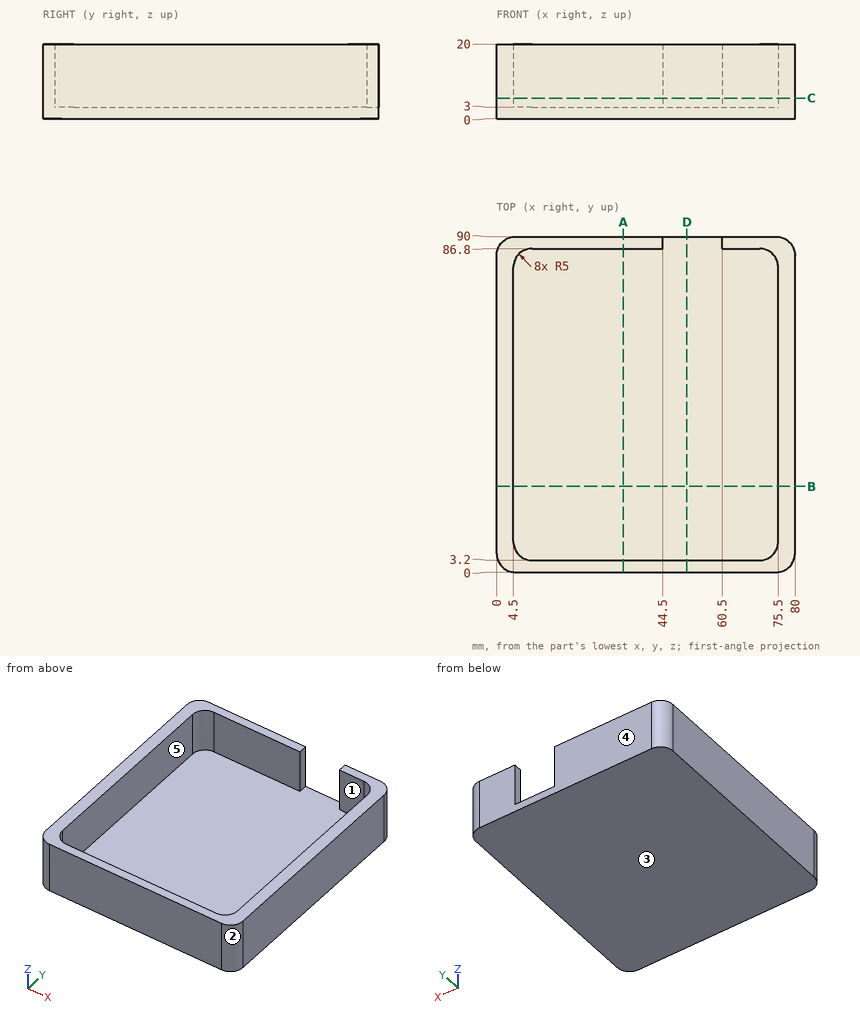
Source: three-view drawing plus pictorial views. Frame: mm from the lowest corner of the part. A direction names the side the tool comes from. Coordinates: 2 decimals unless noted, no trailing zeros. Loops run counter-clockwise (first coordinate to the right, second up) from the corner with the lowest first, then second, coordinate; pieces in that order, holes last. Notation, with made-up numbers: (59, 34) - (64, 34) arc R25 cw to (64, 59) - close; hole circle Ø2 at (9.5, -28). An arc over 180 degrees is marked (long way). One line per item, written item: value. Start each with the question number.
1. Section A-A (x = 34). Return the cut outline in (y, z), and give its area (3 significant figures).
2. Section D-D (x = 51). Return the cut outline in (y, z).
3. Mould query, pull axis Y, two halves, no side actions, for the marked faces 1, 2 and 3. Classes: pulls with the +Y half, pulls with the -Y half, needs draft (parallel to the pull), parting line crosses it, or undercut.
4. Set-up query: the marked faces 4 and 5. Return all of +Z, -Z, +X, -X, +Y, -Y with unobstructed straight access to the full face (end or side cutting, diameter ignored); none if empty.
5. Contact query for flat-ended pins moving along their axis: P1, Ø1, axis at y = 88.5, z = 11.5, coming from the +X side; P2, Ø4, axis at x = 44.5, y = 60, coming from the +Z side; P3, Ø2.5, axis at y = 88.5, z = 7.5, coming from the -X side. Output: stop coordinate, or through.
6. Section B-B (y = 23). Return the cut outline in (x, z).
7. Section C-C (z = 5.5). Return the cut outline in (x, y).
8. Ray query, L1, parallel to Y at x = 16, z = 14; L2, parallel to X at y = 23.5, z = 14.25; L3, parallel to Z at x = 19.5, y = 82. Return the intervals inside material, ascending.
Verdict:
1. outline: (0, 0) - (90, 0) - (90, 20) - (86.8, 20) - (86.8, 3) - (3.2, 3) - (3.2, 20) - (0, 20) - close
1. area: 379 mm2
2. outline: (0, 0) - (90, 0) - (90, 3) - (3.2, 3) - (3.2, 20) - (0, 20) - close
3. face 1: undercut
3. face 2: pulls with the -Y half
3. face 3: needs draft
4. face 4: +Z, -Z, +X, -X, +Y
4. face 5: +Z
5. P1: stops at x = 79
5. P2: stops at z = 3
5. P3: stops at x = 0.53
6. outline: (0, 0) - (80, 0) - (80, 20) - (75.5, 20) - (75.5, 3) - (4.5, 3) - (4.5, 20) - (0, 20) - close
7. outline: (0, 5) arc R5 ccw to (5, 0) - (75, 0) arc R5 ccw to (80, 5) - (80, 85) arc R5 ccw to (75, 90) - (60.5, 90) - (60.5, 86.8) - (70.5, 86.8) arc R5 cw to (75.5, 81.8) - (75.5, 8.2) arc R5 cw to (70.5, 3.2) - (9.5, 3.2) arc R5 cw to (4.5, 8.2) - (4.5, 81.8) arc R5 cw to (9.5, 86.8) - (44.5, 86.8) - (44.5, 90) - (5, 90) arc R5 ccw to (0, 85) - close
8. L1: y = 0 to 3.2, 86.8 to 90
8. L2: x = 0 to 4.5, 75.5 to 80
8. L3: z = 0 to 3
